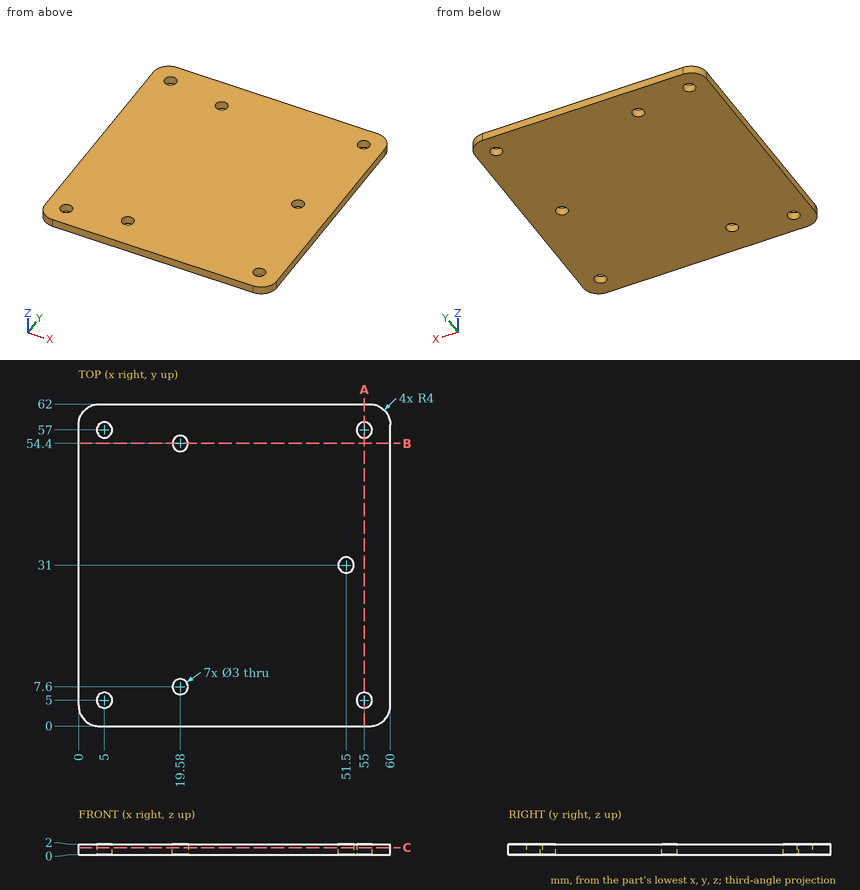
Answer from the drawing. Dimensions are ordinates in mm from the lowest x, y and z of the part. Give positions to 0.01 mm unless a question says otherwise; leave off trailing zeros. Loops run counter-clockwise (first coordinate to the right, second up) from the corner with the lowest first, then second, coordinate; pieces in that order, holes last. Notation, with made-up numbers: (30, 69.25) -> (50, 69.25) arc R14 ccw to (50, 82.25) -> close; hole circle Ø3 at (77, 48.25). An arc over 180 degrees is marked (long way). Answer as CSV lines item,"result".
Item 1: Find section A-A on x = 55. Give the vertices of the cut face in (y, z), plus the area to 3 significant figures.
Returned:
outline,"(0, 0) -> (3.5, 0) -> (3.5, 2) -> (0, 2) -> close; (6.5, 0) -> (55.5, 0) -> (55.5, 2) -> (6.5, 2) -> close; (58.5, 0) -> (62, 0) -> (62, 2) -> (58.5, 2) -> close"
area,"112 mm²"
Item 2: Consider line 1 (Y direction, x = 5, z = 0.4); line 2 (Y direction, x = 19.58, z = 1.1); line 3 (X direction, y = 4.5, z = 1.7). Determine where each line is inside the solid, lowest interval first. Write a range as [from, to].
Returned:
line 1,"y = [0, 3.5], [6.5, 55.5], [58.5, 62]"
line 2,"y = [0, 6.1], [9.1, 52.9], [55.9, 62]"
line 3,"x = [0, 3.59], [6.41, 53.59], [56.41, 60]"
Item 3: Find section B-B on y = 54.4. Give the vertices of the cut face in (x, z), plus the area to 3 significant figures.
Returned:
outline,"(0, 0) -> (18.08, 0) -> (18.08, 2) -> (0, 2) -> close; (21.08, 0) -> (60, 0) -> (60, 2) -> (21.08, 2) -> close"
area,"114 mm²"
Item 4: Find section C-C on z = 1.35. Give the vertices of the cut face in (x, y).
Returned:
outline,"(0, 4) arc R4 ccw to (4, 0) -> (56, 0) arc R4 ccw to (60, 4) -> (60, 58) arc R4 ccw to (56, 62) -> (4, 62) arc R4 ccw to (0, 58) -> close; hole circle Ø3 at (5, 5); hole circle Ø3 at (5, 57); hole circle Ø3 at (19.58, 7.6); hole circle Ø3 at (19.58, 54.4); hole circle Ø3 at (51.5, 31); hole circle Ø3 at (55, 5); hole circle Ø3 at (55, 57)"
